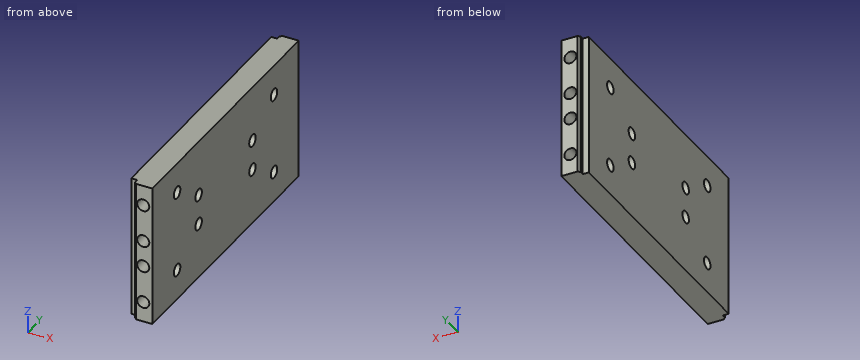
Autodesk Inventor part; units mm, degrees
ref_plane "YZ Plane" through (0, 0, 0) normal (1, 0, 0) x (0, 1, 0)
ref_plane "XZ Plane" through (0, 0, 0) normal (0, 1, 0) x (-1, 0, 0)
ref_plane "XY Plane" through (0, 0, 0) normal (0, 0, 1) x (1, 0, 0)
sketch "Sketch1" plane through (0, 0, 0) normal (0, 0, 1) x (1, 0, 0)
  line L0 (0.0233, 9.5241) -> (9.0233, 9.5241)
  line L1 (0.0233, 9.5241) -> (0.0233, 6.5241)
  line L2 (0.0233, 6.5241) -> (-2.9767, 6.5241)
  line L3 (-2.9767, 6.5241) -> (-2.9767, -123.4759)
  line L4 (-2.9767, -123.4759) -> (0.0233, -123.4759)
  line L5 (0.0233, -123.4759) -> (0.0233, -126.4759)
  line L6 (0.0233, -126.4759) -> (9.0233, -126.4759)
  line L7 (9.0233, -126.4759) -> (9.0233, 9.5241)
  dimension "d0" = 9
  dimension "d1" = 3
  dimension "d2" = 3
  dimension "d3" = 130
  dimension "d4" = 3
  dimension "d5" = 9
extrude "Extrusion1" add sketch "Sketch1" along normal blind 70
sketch "Sketch2" plane through (0.0233, 9.5241, 0) normal (0, 1, 0) x (1, 0, 0)
  circle A0 centre (4.5, -10) radius 3
  circle A1 centre (4.5, -28.5) radius 3
  circle A2 centre (4.5, -41.5) radius 3
  circle A3 centre (4.5, -60) radius 3
  line L0 (9, -70) -> (0, -70)
  line L1 (9, 0) -> (0, 0)
  line L2 (0, 0) -> (0, -70)
  point P0 (-0.0233, 0)
  dimension "d8" = 6
  dimension "d9" = 6
  dimension "d10" = 6
  dimension "d11" = 6
  dimension "d12" = 10
  dimension "d16" = 10
  dimension "d18" = 4.5
  dimension "d19" = 4.5
  dimension "d20" = 4.5
  dimension "d21" = 4.5
  dimension "d135" = 28.5
  dimension "d136" = 28.5
sketch "Sketch3" plane through (0.0233, -126.4759, 0) normal (0, -1, 0) x (1, 0, 0)
  circle A0 centre (4.5, 10) radius 3
  circle A1 centre (4.5, 28.5) radius 3
  circle A2 centre (4.5, 41.5) radius 3
  circle A3 centre (4.5, 60) radius 3
  line L0 (0, 70) -> (9, 70)
  line L1 (0, 0) -> (9, 0)
  line L2 (0, 0) -> (0, 70)
  point P0 (-0.0233, 0)
  dimension "d38" = 6
  dimension "d39" = 6
  dimension "d40" = 6
  dimension "d41" = 6
  dimension "d42" = 10
  dimension "d43" = 10
  dimension "d46" = 4.5
  dimension "d47" = 4.5
  dimension "d48" = 4.5
  dimension "d49" = 4.5
  dimension "d137" = 28.5
  dimension "d138" = 28.5
sketch "Sketch4" plane through (-2.9767, -123.4759, 0) normal (-1, 0, 0) x (0, 0, 1)
  circle A0 centre (15, 110) radius 3
  circle A1 centre (27.5, 90) radius 3
  circle A2 centre (42.5, 90) radius 3
  circle A3 centre (55, 110) radius 3
  line L0 (0, 133) -> (70, 133)
  line L1 (0, 130) -> (0, 0)
  line L2 (70, 130) -> (70, 0)
  line L3 (70, -3) -> (70, 133)
  line L4 (70, 65) -> (60.0222, 65)
  circle A4 centre (15, 20) radius 3
  circle A5 centre (27.5, 40) radius 3
  circle A6 centre (42.5, 40) radius 3
  circle A7 centre (55, 20) radius 3
  circle A8 centre (15, 110) radius 5.125
  circle A9 centre (27.5, 90) radius 5.125
  circle A10 centre (42.5, 90) radius 5.125
  circle A11 centre (55, 110) radius 5.125
  circle A12 centre (15, 20) radius 5.125
  circle A13 centre (27.5, 40) radius 5.125
  circle A14 centre (42.5, 40) radius 5.125
  circle A15 centre (55, 20) radius 5.125
  circle A16 centre (35, 65) radius 3
  line L5 (35, 65) -> (35, 82.0143)
  circle A17 centre (60, 82.0143) radius 3
  circle A18 centre (45, 82.0143) radius 3
  circle A19 centre (10, 86.2004) radius 3
  point P0 (0, 123.4759)
  dimension "d52" = 6
  dimension "d53" = 6
  dimension "d54" = 6
  dimension "d55" = 6
  dimension "d56" = 23
  dimension "d57" = 43
  dimension "d58" = 43
  dimension "d59" = 23
  dimension "d60" = 15
  dimension "d61" = 15
  dimension "d66" = 10.25
  dimension "d67" = 10.25
  dimension "d68" = 10.25
  dimension "d69" = 10.25
  dimension "d70" = 10.25
  dimension "d71" = 10.25
  dimension "d72" = 10.25
  dimension "d73" = 10.25
  dimension "d76" = 6
  dimension "d77" = 6
  dimension "d78" = 6
  dimension "d79" = 10
  dimension "d80" = 15
  dimension "d83" = 6
  dimension "d85" = 10
  dimension "d133" = 12.5
  dimension "d134" = 12.5
extrude "Extrusion5" cut sketch "Sketch4" against normal blind 21 contours A0 | A1 | A2 | A3 | A4 | A5 | A6 | A7
hole "Agujero1" at (4.5233, 9.5241, 10) at (4.5233, 9.5241, 28.5) at (4.5233, 9.5241, 41.5) at (4.5233, 9.5241, 60) direction (0, -1, 0) diameter 6 depth 15 tip angle 118
hole "Agujero2" at (4.5233, -126.4759, 10) at (4.5233, -126.4759, 28.5) at (4.5233, -126.4759, 41.5) at (4.5233, -126.4759, 60) direction (0, 1, 0) diameter 6 depth 15 tip angle 118
thread "Rosca9"
thread "Rosca10"
thread "Rosca11"
thread "Rosca12"
thread "Rosca13"
thread "Rosca14"
thread "Rosca15"
thread "Rosca16"
chamfer "Chaflán1" distance 1 angle 45 2 edges at (0.0233, 9.5241, 35) (0.0233, -126.4759, 35)
equation "\"d16\" = d12"
equation "\"d136\" = d135"
equation "\"d43\" = d42"
equation "\"d138\" = d137"
properties part number "Vertical Vìnculo Cabezal" material "Aluminum 6061"
Build history of the part. All positions in model axes, mm. Round coordinates to 2 decimals unless told otherwise and drop trailing zeros. Write each loop counter-clockwise with the first axis right and the second up, starting at its lowest first coordinate (ties: lowest second). Pieces come first, ordered by that corner, then holes. Notation, with made-up numbers: M -19,80 L 8,80 A12 cw 8,90 Z; hole C 76,-9 d1. An arc over 180 degrees is marked long. Answer in a Markdown table with one row per item.
1. Saw through at A-A (z = 55). List the corners of the cut face in (x, y).
Geometry check:
| item | result |
|---|---|
| outline | M -2.98,-123.48 L 0.02,-123.48 L 0.02,-125.48 L 1.02,-126.48 L 9.02,-126.48 L 9.02,-106.48 L -2.98,-106.48 Z; M -2.98,-100.48 L 9.02,-100.48 L 9.02,-16.48 L -2.98,-16.48 Z; M -2.98,-10.48 L 9.02,-10.48 L 9.02,9.52 L 1.02,9.52 L 0.02,8.52 L 0.02,6.52 L -2.98,6.52 Z |
2. Flat gauge pins, fed straight in: P1, Ø1.5, axis at x = -1, z = 22, coming from the -Y side; P2, Ø0.6, axis at y = -124.5, z = 52, coming from the -X side; P3, Ø5.5, axis at x = 4.52, z = 10, coming from the +Y side. Where does each tip first touch, or does it go through?
Geometry check:
| item | result |
|---|---|
| P1 | y = -123.48 |
| P2 | x = 0.02 |
| P3 | y = -5.62 |
3. Probe L1, parallel to Y at x = 5.5, z = 42; L2, parallel to Z at x = 5.5, y = -106; L3, parallel to Z at x = 2.5, y = -1.5 (3 decimals). List the from-to ranges inside material, lowest first. Write a range as [from, to].
Geometry check:
| item | result |
|---|---|
| L1 | [-110.33, -86.43], [-80.52, -36.43], [-30.52, -6.62] |
| L2 | [0, 13.38], [16.62, 53.38], [56.62, 70] |
| L3 | [0, 7.785], [12.215, 26.285], [30.715, 39.285], [43.715, 57.785], [62.215, 70] |
4. Saw through at B-B (x = 3.25). State how many separate pieces and enclosed holes the cut face has, and give its area (3 significant figures).
Geometry check:
| item | result |
|---|---|
| separate pieces | 1 |
| enclosed holes | 8 |
| area | 8,610 mm2 |
